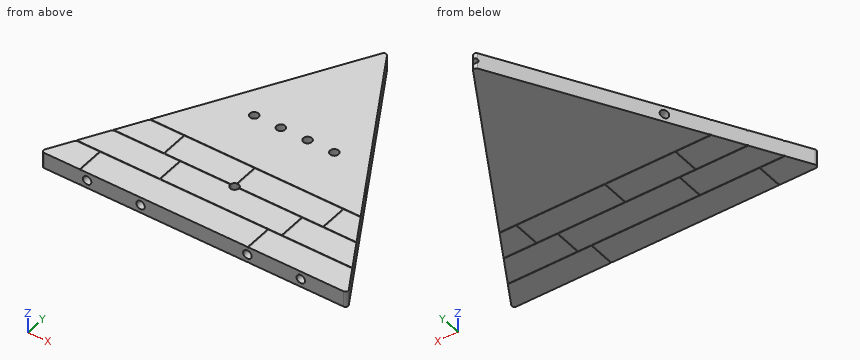
```python
from build123d import *

# Parameters (mm, degrees)
F3_DEPTH       = 6
F4_W           = 32.6863850343
F4_H           = 10.1006624426
F4_W_2         = 25.8918322674
F5_DEPTH       = 0.15
F6_W           = 25.8918322674
F6_H           = 10.1006624426
F6_W_2         = 45.1567518413
F6_W_3         = 32.6863850343
F7_DEPTH       = 0.15
F8_R           = 1.6
F9_DEPTH       = 5
F11_R          = 1.05
F12_DEPTH      = 5
F12_DEPTH_BACK = 0.501
F13_R          = 1.6
F14_DEPTH      = 5
F15_R          = 1.6
F16_DEPTH      = 5
F17_R          = 1.6
F18_DEPTH      = 5


with BuildPart() as f3:
    # F2 (on Top) → F3 (new body)
    with BuildSketch(Plane.XY):
        with BuildLine():
            ThreePointArc((0.8660254038, 98.5), (0, 99), (-0.8660254038, 98.5))
            Line((-0.8660254038, 98.5), (-56.8690015152, 1.5))
            ThreePointArc((-56.8690015152, 1.5), (-56.8690015152, 0.5), (-56.0029761114, 0))
            Line((-56.0029761114, 0), (56.0029761114, 0))
            ThreePointArc((56.0029761114, 0), (56.8690015152, 0.5), (56.8690015152, 1.5))
            Line((56.8690015152, 1.5), (0.8660254038, 98.5))
        make_face()
    extrude(amount=F3_DEPTH)

    # F4 (on face) → F5 (cut)
    with BuildSketch(Plane.XY.offset(6)):
        Polygon((39.6628161091, 31.3019873277), (39.3741409745, 31.8019873277), (0, 31.8019873277), (0, 20.7013248852), (25.1688986466, 20.7013248852), (25.1688986466, 10.6006624426), (0, 10.6006624426), (0, 10.1006624426), (20.1229155064, 10.1006624426), (20.1229155064, 0), (20.6229155064, 0), (20.6229155064, 10.1006624426), (51.9034067387, 10.1006624426), (51.6147316042, 10.6006624426), (25.6688986466, 10.6006624426), (25.6688986466, 20.7013248852), (45.7831114239, 20.7013248852), (45.4944362893, 21.2013248852), (33.4497465572, 21.2013248852), (33.4497465572, 31.3019873277), align=None)
        with Locations((16.60655404, 26.2516561065)):
            Rectangle(F4_W, F4_H, mode=Mode.SUBTRACT)
        Polygon((0, 20.7013248852), (0, 31.8019873277), (-39.3741409745, 31.8019873277), (-39.6628161091, 31.3019873277), (-26.6284707446, 31.3019873277), (-26.6284707446, 21.2013248852), (-45.4944362893, 21.2013248852), (-45.7831114239, 20.7013248852), (-20.4878531947, 20.7013248852), (-20.4878531947, 10.6006624426), (-51.6147316042, 10.6006624426), (-51.9034067387, 10.1006624426), (-42.7899323404, 10.1006624426), (-42.7899323404, 0), (-42.2899323404, 0), (-42.2899323404, 10.1006624426), (0, 10.1006624426), (0, 10.6006624426), (-19.9878531947, 10.6006624426), (-19.9878531947, 20.7013248852), align=None)
        with Locations((-13.1825546109, 26.2516561065)):
            Rectangle(F4_W_2, F4_H, mode=Mode.SUBTRACT)
    extrude(amount=-F5_DEPTH, mode=Mode.SUBTRACT)

    # F6 (on face) → F7 (cut)
    with BuildSketch(Plane.XY):
        Polygon((-51.9034067387, 10.1006624426), (-42.7899323404, 10.1006624426), (-42.7899323404, 0), (-42.2899323404, 0), (-42.2899323404, 10.1006624426), (20.1229155064, 10.1006624426), (20.1229155064, 0), (20.6229155064, 0), (20.6229155064, 10.1006624426), (51.9034067387, 10.1006624426), (51.6147316042, 10.6006624426), (25.6688986466, 10.6006624426), (25.6688986466, 20.7013248852), (45.7831114239, 20.7013248852), (45.4944362893, 21.2013248852), (33.4497465572, 21.2013248852), (33.4497465572, 31.3019873277), (39.6628161091, 31.3019873277), (39.3741409745, 31.8019873277), (-39.3741409745, 31.8019873277), (-39.6628161091, 31.3019873277), (-26.6284707446, 31.3019873277), (-26.6284707446, 21.2013248852), (-45.4944362893, 21.2013248852), (-45.7831114239, 20.7013248852), (-20.4878531947, 20.7013248852), (-20.4878531947, 10.6006624426), (-51.6147316042, 10.6006624426), align=None)
        with Locations((-13.1825546109, 26.2516561065)):
            Rectangle(F6_W, F6_H, mode=Mode.SUBTRACT)
        with Locations((2.5905227259, 15.6509936639)):
            Rectangle(F6_W_2, F6_H, mode=Mode.SUBTRACT)
        with Locations((16.60655404, 26.2516561065)):
            Rectangle(F6_W_3, F6_H, mode=Mode.SUBTRACT)
    extrude(amount=F7_DEPTH, mode=Mode.SUBTRACT)

    # F8 (on face) → F9 (cut)
    with BuildSketch(Plane.XY.offset(6)):
        with BuildLine():
            ThreePointArc((1.5937095858, 20.7013248852), (1.6084409724, 20.8259392813), (1.6133615229, 20.9513248852))
            ThreePointArc((1.6133615229, 20.9513248852), (1.6084409724, 21.076710489), (1.5937095858, 21.2013248852))
            ThreePointArc((1.5937095858, 21.2013248852), (1.1447323728, 22.0826957351), (0.2633615229, 22.5316729481))
            ThreePointArc((0.2633615229, 22.5316729481), (0.0133615229, 22.5513248852), (-0.2366384771, 22.5316729481))
            ThreePointArc((-0.2366384771, 22.5316729481), (-1.118009327, 22.0826957351), (-1.5669865401, 21.2013248852))
            ThreePointArc((-1.5669865401, 21.2013248852), (-1.5866384771, 20.9513248852), (-1.5669865401, 20.7013248852))
            ThreePointArc((-1.5669865401, 20.7013248852), (0.0133615229, 19.3513248852), (1.5937095858, 20.7013248852))
        make_face()
        with Locations((5, 51.8019873277)):
            Circle(F8_R)
        with Locations((-5, 51.8019873277)):
            Circle(F8_R)
        with Locations((15, 51.8019873277)):
            Circle(F8_R)
        with Locations((-15, 51.8019873277)):
            Circle(F8_R)
    extrude(amount=-F9_DEPTH, mode=Mode.SUBTRACT)

    # F11 (on 3pt) → F12 (cut, two sides)
    with BuildSketch(Plane.XZ.offset(-98.5)) as f12_sk:
        with Locations((0, 3)):
            Circle(F11_R)
    extrude(amount=F12_DEPTH, mode=Mode.SUBTRACT)
    extrude(f12_sk.sketch, amount=-F12_DEPTH_BACK, mode=Mode.SUBTRACT)

    # F13 (on face) → F14 (cut)
    with BuildSketch(Plane.XZ):
        with Locations((-40, 3)):
            Circle(F13_R)
        with Locations((-20, 3)):
            Circle(F13_R)
        with Locations((20, 3)):
            Circle(F13_R)
        with Locations((40, 3)):
            Circle(F13_R)
    extrude(amount=-F14_DEPTH, mode=Mode.SUBTRACT)

    # F15 (on face) → F16 (cut)
    with BuildSketch(Plane(origin=(43.3012701892, 25, 0), x_dir=(-0.5, 0.8660254038, 0), z_dir=(0.8660254038, 0.5, 0))):
        with Locations((22.8645373481, 3)):
            Circle(F15_R)
    extrude(amount=-F16_DEPTH, mode=Mode.SUBTRACT)

    # F17 (on face) → F18 (cut)
    with BuildSketch(Plane(origin=(-43.3012701892, 25, 0), x_dir=(-0.5, -0.8660254038, 0), z_dir=(-0.8660254038, 0.5, 0))):
        with Locations((-22.8645373481, 3)):
            Circle(F17_R)
    extrude(amount=-F18_DEPTH, mode=Mode.SUBTRACT)


solid = f3.part
```
CAD build for the part. Positions are in the model's coordinates, mm. Round coordinates to 2 decimals unless told otherwise and drop trailing zeros. Write each loop counter-clockwise with the first axis right and the second up, starting at its lowest first coordinate (ties: lowest second). Pieces come first, ordered by that corner, then holes. Notation, with made-up numbers: M 23.25,78.25 L 53.25,78.25 A13 ccw 53.25,102.25 Z; hole C 49,21 d6. An arc over 180 degrees is marked long. One line per question, with ' | ' between items.
1. Cut at C-C on y = 14. Write the cut outline in (x, z).
Working result:
outline: M -49.65,0 L -20.49,0 L -20.49,0.15 L -19.99,0.15 L -19.99,0 L 25.17,0 L 25.17,0.15 L 25.67,0.15 L 25.67,0 L 49.65,0 L 49.65,6 L 25.67,6 L 25.67,5.85 L 25.17,5.85 L 25.17,6 L -19.99,6 L -19.99,5.85 L -20.49,5.85 L -20.49,6 L -49.65,6 Z
2. Cut at A-A on y = 26. Write the cut outline in (x, z), and give its area (3 significant figures).
Working result:
outline: M -42.72,0 L -26.63,0 L -26.63,0.15 L -26.13,0.15 L -26.13,0 L -0.24,0 L -0.24,0.15 L 0.26,0.15 L 0.26,0 L 32.95,0 L 32.95,0.15 L 33.45,0.15 L 33.45,0 L 42.72,0 L 42.72,6 L 33.45,6 L 33.45,5.85 L 32.95,5.85 L 32.95,6 L 0.26,6 L 0.26,5.85 L -0.24,5.85 L -0.24,6 L -26.13,6 L -26.13,5.85 L -26.63,5.85 L -26.63,6 L -42.72,6 Z | area: 512 mm2
3. Pin check, flat tips, straight feed: pin 1 Ø3 at (x, z) = (-40, 3) entering from +Y; pin 2 Ø2 at (y, z) = (12.5, 4.5) entering from +X; pin 3 Ø1 at (y, z) = (16, 4.5) entering from +X. Stop position of each tip, or through.
Working result:
pin 1: y = 33.32 | pin 2: x = 51.1 | pin 3: x = 48.79
4. Cut at D-D on y = 56. Write the cut outline in (x, z).
Working result:
outline: M -25.4,0 L 25.4,0 L 25.4,6 L -25.4,6 Z
5. Probe L1, parallel to Z at x = 40, y = 3; L2, parallel to Y at x = -15.5, z = 4.75; L3, parallel to Y at x = 34, z = 3. List the from-to ranges inside material, lowest first. Write a range as from..to.
Working result:
L1: 0..1.4, 4.6..6 | L2: 0..50.28, 53.32..73.15 | L3: 0..41.11
